For this review, take the finished solid that the model builds, in its own axes (mm). A direction names the side the tool comes from. Round coordinates to 2 decimals unless told otherwise and drop trailing zeros. Put each result on its own line as item: value.
Autodesk Inventor part; units mm, degrees
ref_plane "YZ Plane" through (0, 0, 0) normal (1, 0, 0) x (0, 1, 0)
ref_plane "XZ Plane" through (0, 0, 0) normal (0, 1, 0) x (-1, 0, 0)
ref_plane "XY Plane" through (0, 0, 0) normal (0, 0, 1) x (1, 0, 0)
sketch "Sketch1" plane through (0, 0, 0) normal (0, 0, 1) x (1, 0, 0)
  line L0 (0, 0) -> (-19.2, 0)
  line L1 (-19.2, 0) -> (-20.2, 35)
  line L2 (-20.2, 35) -> (-25.2, 35)
  arc A0 (-3, 135) -> (-25.2, 35) centre (174.6359, 43.1006) ccw
  line L3 (-3, 135) -> (0, 135)
  line L4 (0, 135) -> (0, 0)
  dimension "d0" = 19.2
  dimension "d1" = 35
  dimension "d2" = 1
  dimension "d3" = 5
  dimension "d4" = 200
  dimension "d5" = 100
  dimension "d6" = 3
revolve "Revolution1" add sketch "Sketch1" angle 360 about axis through (0, 135, 0) along (0, -1, 0)
fillet "Fillet1" radius 4 1 edges at (3, 135, 0)
fillet "Fillet2" radius 3 1 edges at (25.2, 35, 0)
equation "\"BendRadius\" = Thickness"
equation "\"BendReliefWidth\" = Thickness"
equation "\"BendReliefDepth\" = 0.5 * Thickness"
equation "\"CornerReliefSize\" = 4 * Thickness"
equation "\"MinimumRemnant\" = 2 * Thickness"
equation "\"TransitionRadius\" = BendRadius"
equation "\"JacobiRadiusSize\" = BendRadius"
equation "\"GapSize\" = Thickness"
properties part number "noseconefairing"
(1) For faces 1 (the face through (-18.8, 17.7, 5.9)), 2 (the face through (0, 0, 0)), list the 3-axis set-ups (+Z, -Z, +X, -X, +Y, -Y) from which the entire face can be reached by the end or side of a thin tool; tool diameter is ignored.
A:
face 1: -Y
face 2: +Z, -Z, +X, -X, -Y
(2) To check wall thickness, follow L1, parallel to X at y = 104, z = 0; L2, parallel to Y at x = 1, z = -3.5; L3, parallel to Y at x = 3.5, z = -0.5. State the ranges of each line that lie inside material, in increasing order.
A:
L1: x = -15.87 to 15.87
L2: y = 0 to 133.54
L3: y = 0 to 133.66
(3) Insertion check: pin 1 Ø4 at (x, y) = (5.5, 85) entering from -Z; pin 2 Ø12 at (x, y) = (-16, 88.5) entering from +Z; pin 3 Ø1 at (y, z) = (69, 7) entering from +X. Each pin has a flat end and moves straight along its axis. Give the tip position at first contact, or say it passes through.
A:
pin 1: stops at z = -20.83
pin 2: stops at z = 17.82
pin 3: stops at x = 22.79
